```python
from build123d import *

# Parameters (mm, degrees)
SKETCH1_R                 = 12.7
BOSS_EXTRUDE1_DEPTH       = 50.8
SKETCH2_R                 = 1.5875
BOSS_EXTRUDE2_DEPTH       = 59.69
F_2_64_TAPPED_HOLE1_D     = 1.778
F_2_64_TAPPED_HOLE1_DEPTH = 12.7
F_2_64_TAPPED_HOLE1_TIP   = 0.53416509


with BuildPart() as part:
    # Sketch1 → Boss-Extrude1 (new body)
    with BuildSketch(Plane.XY):
        with Locations(Location((0, 0, 0), (0, 0, 180))):
            Circle(SKETCH1_R)
    extrude(amount=BOSS_EXTRUDE1_DEPTH)

    # Sketch2 → Boss-Extrude2 (add)
    with BuildSketch(Plane(origin=(0, 0, 0), x_dir=(-1, 0, 0), z_dir=(0, 0, -1))):
        with Locations(Location((0, 0, 0), (0, 0, 180))):
            Circle(SKETCH2_R)
    extrude(amount=BOSS_EXTRUDE2_DEPTH)

    # #2-64 Tapped Hole1
    with Locations(Plane(origin=(0, 0, 0), x_dir=(-1, 0, 0), z_dir=(0, 0, -1))):
        with Locations((-7.62, 7.62), (7.62, 7.62), (7.62, -7.62), (-7.62, -7.62)):
            Hole(F_2_64_TAPPED_HOLE1_D / 2, depth=F_2_64_TAPPED_HOLE1_DEPTH)
            with Locations((0, 0, -(F_2_64_TAPPED_HOLE1_DEPTH + F_2_64_TAPPED_HOLE1_TIP / 2))):  # 118° drill point
                Cone(0, F_2_64_TAPPED_HOLE1_D / 2, F_2_64_TAPPED_HOLE1_TIP, mode=Mode.SUBTRACT)


solid = part.part
```
Work out the finished part from the listing and answer in its coordinate system (mm). A direction names the side the tool comes from. Round coordinates to 2 decimals unless told otherwise and drop trailing zeros. Write each loop counter-clockwise with the first axis right and the second up, starting at its lowest first coordinate (ties: lowest second). Pieces come first, ordered by that corner, then holes.
1) Determine the mould class of faces 3 (the face through (-7.81, 6.75, 6.44)), 4 (the face through (-8.51, -7.58, 6.44)), 5 (the face through (0, 0, 50.8)), 6 (the face through (-5.86, 11.267, 25.044)) for opening direction X: pulls with the +X half, pulls with the -X half, needs draft (parallel to the pull), parting line crosses it, or undercut.
2) A cutting plane is placed at D-D on x = -4.75. Determine the outline of the cut face in (y, z), and give its area (3 significant figures).
3) Consider probe 1 along X at (y, z) = (-7.62, 7.25); probe 2 along X at (y, z) = (7, 2). Determine where each line is inside the solid, lowest interval first.
4) A cutting plane is placed at A-A on x = 0. Determine the outline of the cut face in (y, z).
5) Which of the six approach directions +Z, -Z, +X, -X, +Y, -Y give full straight-line access (tool end or side, diameter ignored) to faces 1 (the face through (0.73, 1.41, -29.43)), 2 (the face through (0, 0, -59.69))?
6) Flat-ended cylindrical pins translate along their axes: P1, Ø2, axis at x = -7.62, y = 7.62, coming from the -Z side; P2, Ø10, axis at y = -0.5, z = -11.5, coming from the -X side; P3, Ø2, axis at x = -4, z = 17, coming from the +Y side. Find the tip coordinate at first contact, or state that the pin passes through.
7) A cutting plane is placed at C-C on z = -5.5. Determine the outline of the cut face in (x, y) (1 decimal), and give its area (3 significant figures).
Entries:
1. face 3: undercut
1. face 4: undercut
1. face 5: needs draft
1. face 6: parting line crosses it
2. outline: (-11.78, 0) - (11.78, 0) - (11.78, 50.8) - (-11.78, 50.8) - close
2. area: 1,200 mm2
3. probe 1: x = -10.16 to -8.51, -6.73 to 6.73, 8.51 to 10.16
3. probe 2: x = -10.6 to -8.26, -6.98 to 6.98, 8.26 to 10.6
4. outline: (-12.7, 0) - (-1.59, 0) - (-1.59, -59.69) - (1.59, -59.69) - (1.59, 0) - (12.7, 0) - (12.7, 50.8) - (-12.7, 50.8) - close
5. face 1: -Z
5. face 2: -Z, +X, -X, +Y, -Y
6. P1: stops at z = 0
6. P2: stops at x = -1.59
6. P3: stops at y = 12.34
7. outline: circle Ø3.2 at (0, 0)
7. area: 7.92 mm2
